Geometry: final body of the model. Coordinates: model frame, mm. Give positions to 0.01 mm unless a question says otherwise; leave off trailing zeros. Order: outer loops, then holes, each group sorted by start corner. A loop starts at its lowest first (then second) coordinate and runs counter-clockwise, first axis right, second up. Notation, with made-up numbers: (46.5, 39) -> (86.5, 39) arc R19 ccw to (86.5, 60) -> close; hole circle Ø3 at (79.25, 4.5). An arc over 180 degrees is marked (long way). Write item = value, one per line.
```python
from build123d import *

# Parameters (mm, degrees)
F1_DEPTH = 25
F2_R     = 1.5875
F3_DEPTH = 25


with BuildPart() as f1:
    # F0 (on Front) → F1 (new body)
    with BuildSketch(Plane.XZ):
        with BuildLine():
            ThreePointArc((-17.7535207776, 10.25), (-18.9395304165, 7.8450103635), (-19.8014794389, 5.3057904246))
            add(Edge.make_bspline(
                [(-19.8014794389, 5.3057904246), (-20.454122155, 2.8700946489), (-19.9763700286, -0.7893865531), (-18.8355536126, -5.0469713795)],
                knots=[0, 0, 0, 0, 10.3977252163, 10.3977252163, 10.3977252163, 10.3977252163], degree=3))
            ThreePointArc((-18.8355536126, -5.0469713795), (-19.3331747968, 2.5452607483), (-16.8874953738, 9.75))
            Line((-16.8874953738, 9.75), (-17.7535207776, 10.25))
        make_face()
        with BuildLine():
            add(Edge.make_bspline(
                [(19.8014794389, 5.3057904246), (20.454122155, 2.8700946489), (19.9763700286, -0.7893865531), (18.8355536126, -5.0469713795)],
                knots=[0, 0, 0, 0, 10.3977252163, 10.3977252163, 10.3977252163, 10.3977252163], degree=3))
            ThreePointArc((19.8014794389, 5.3057904246), (2.6757869405, 20.3246196582), (-17.7535207776, 10.25))
            Line((-17.7535207776, 10.25), (-16.8874953738, 9.75))
            ThreePointArc((-16.8874953738, 9.75), (5.0469713795, 18.8355536126), (19.5, 0))
            ThreePointArc((19.5, 0), (19.3331747968, -2.5452607483), (18.8355536126, -5.0469713795))
        make_face()
        with BuildLine():
            ThreePointArc((-16.8874953738, -9.75), (0, -19.5), (16.8874953738, -9.75))
            ThreePointArc((16.8874953738, -9.75), (18.015650884, -7.4623269311), (18.8355536126, -5.0469713795))
            ThreePointArc((18.8355536126, -5.0469713795), (19.3331747968, -2.5452607483), (19.5, 0))
            ThreePointArc((19.5, 0), (5.0469713795, 18.8355536126), (-16.8874953738, 9.75))
            ThreePointArc((-16.8874953738, 9.75), (-19.3331747968, 2.5452607483), (-18.8355536126, -5.0469713795))
            ThreePointArc((-18.8355536126, -5.0469713795), (-18.015650884, -7.4623269311), (-16.8874953738, -9.75))
        make_face()
        with BuildLine():
            add(Edge.make_bspline(
                [(-16.8874953738, -9.75), (-15.9041162308, -11.4532626388), (-15.0411330668, -13.0764351646), (-14.2892263879, -14.6992519958)],
                knots=[0, 0, 0, 0, 6.1017074107, 6.1017074107, 6.1017074107, 6.1017074107], degree=3))
            ThreePointArc((-14.2892263879, -14.6992519958), (-0.3862841846, -20.4963602751), (13.7252177136, -15.2272255751))
            Line((13.7252177136, -15.2272255751), (16.8874953738, -9.75))
            ThreePointArc((16.8874953738, -9.75), (0, -19.5), (-16.8874953738, -9.75))
        make_face()
        with BuildLine():
            Line((-10, -40), (10, -40))
            add(Edge.make_bspline(
                [(14.2892263879, -14.6992519958), (11.2180568693, -21.327661778), (10, -27.950137429), (10, -40)],
                knots=[6.1017074107, 6.1017074107, 6.1017074107, 6.1017074107, 31.0241856061, 31.0241856061, 31.0241856061, 31.0241856061], degree=3))
            ThreePointArc((14.2892263879, -14.6992519958), (14.0097094404, -14.9658959436), (13.7252177136, -15.2272255751))
            ThreePointArc((13.7252177136, -15.2272255751), (-0.3862841846, -20.4963602751), (-14.2892263879, -14.6992519958))
            add(Edge.make_bspline(
                [(-14.2892263879, -14.6992519958), (-11.2180568693, -21.327661778), (-10, -27.950137429), (-10, -40)],
                knots=[6.1017074107, 6.1017074107, 6.1017074107, 6.1017074107, 31.0241856061, 31.0241856061, 31.0241856061, 31.0241856061], degree=3))
        make_face()
        with BuildLine():
            ThreePointArc((13.7252177136, -15.2272255751), (14.0097094404, -14.9658959436), (14.2892263879, -14.6992519958))
            add(Edge.make_bspline(
                [(16.8874953738, -9.75), (15.9041162308, -11.4532626388), (15.0411330668, -13.0764351646), (14.2892263879, -14.6992519958)],
                knots=[0, 0, 0, 0, 6.1017074107, 6.1017074107, 6.1017074107, 6.1017074107], degree=3))
            Line((16.8874953738, -9.75), (13.7252177136, -15.2272255751))
        make_face()
    extrude(amount=F1_DEPTH)

    # F2 (on face) → F3 (cut)
    with BuildSketch(Plane.XZ.offset(25)):
        Circle(F2_R)
    extrude(amount=-F3_DEPTH, mode=Mode.SUBTRACT)


solid = f1.part
```
1) Section query B-B (z = 16). Output: boundary loops of the cut face in (x, y), plus the area to 3 significant figures.
Check sheet entries:
outline = (-12.82, -25) -> (12.82, -25) -> (12.82, 0) -> (-12.82, 0) -> close
area = 641 mm²
2) First-contact query: P1, Ø3, axis at x = 8.5, y = -6, coming from the +Z side; P2, Ø1, axis at x = -10.5, y = -15, coming from the +Z side; P3, Ø10, axis at y = -3, z = -11, coming from the +X side. Flat tips, straight axial feed; report the tip coordinate or a pass-through.
Check sheet entries:
P1 = 19.27
P2 = 17.9
P3 = 18.55
3) Line query: line 1 (Z direction, x = 0, y = -21.25); line 2 (X direction, y = -2.25, z = -13); line 3 (X direction, y = -5.5, z = -22). Output: solid intervals per line, ascending. Write a range as from..to.
Check sheet entries:
line_1 = -40..-1.59, 1.59..20.5
line_2 = -15.12..15.12
line_3 = -11.69..11.69
4) Mould query, pull axis Z, two halves, no side actions, for faces 1 (the face through (0, -25, -9)), 2 (the face through (-0.34, -12.68, -1.55)), 3 (the face through (18, -12.3, -7.5)). Classes: +Z half, -Z half, draft (parallel to the pull), parting line (faces both ways), or undercut.
Check sheet entries:
face_1 = draft
face_2 = undercut
face_3 = -Z half
5) Section query A-A (x = 0). Output: boundary loops of the cut face in (y, z), plus the area to 3 significant figures.
Check sheet entries:
outline = (-25, -40) -> (0, -40) -> (0, -1.59) -> (-25, -1.59) -> close; (-25, 1.59) -> (0, 1.59) -> (0, 20.5) -> (-25, 20.5) -> close
area = 1,430 mm²
